Geometry check sheet. Reference: the model listing, model coordinates, mm. A direction names the side the tool comes from. Round coordinates to 2 decimals unless told otherwise and drop trailing zeros. Loops run counter-clockwise (first coordinate to the right, second up) from the corner with the lowest first, then second, coordinate; pieces in that order, holes last. Notation, with made-up numbers: (-5, 82) -> (2, 82) arc R19 ccw to (2, 101) -> close; hole circle Ø5 at (-29.5, 62.25). An arc over 180 degrees is marked (long way). Use a Markdown table: item, result. Add a question column.
Q1. Sectioned sample at A-A, the plane z = 50. Enter the section's corners in (x, y).
Q2. Gauge pin test, flat ends, axial feed: P1, Ø12, axis at x = 16.5, y = -13, coming from the -Z side; P2, Ø12, axis at x = 10.5, y = -11, coming from the +Z side; P3, Ø3.5, axis at x = 19.18, z = 50, coming from the +Y side; P4, Ø8, axis at x = 8.5, z = 10, coming from the -Y side. Record the tip position at first contact, or that the pin passes through.
Q3. Sectioned sample at C-C, the plane y = 3.75. Give the number of separate pieces and of enclosed holes in the cut face, then the cut area to 3 significant figures.
Q4. Set-up check for faces 4 (the face through (21.53, 2.33, 9.69)), 5 (the face through (20.37, 5.46, 29.73)), 6 (the face through (12, -12, 40)), 7 (the face through (12, 0, 10)): record each of +Z, -Z, +X, -X, +Y, -Y from which the full face is reachable in a straight line by a thin tool's end or side.
Q5. Release check for a two-part mould opening along Z. For faces 1 (the face through (3.64, 2.33, 48.12)), 2 (the face through (12, -2, 19)), 3 (the face through (20.37, 5.46, 55.4)) record: released by +Z, released by -Z, zero draft, split by the parting line, or undercut.
Q6. Material ranges on L1, parallel to Z at x = 19.18, y = 5.4; L2, parallel to X at y = 6.4, z = 10; L3, parallel to X at y = 5.25, z = 10, recorded low to high.
Q7. Sectioned sample at B-B, the plane y = -15.75. Enter the section's corners in (x, z).
```python
from build123d import *

# Parameters (mm, degrees)
EXTRUDE_1_DEPTH             = 60
HOLE_WIZARD_M41_D           = 4.5
HOLE_WIZARD_M41_CSINK_D     = 9.4
HOLE_WIZARD_M41_CSINK_ANGLE = 90
EXTRUDE_2_DEPTH             = 24.26
CHAMFER_1_SIZE              = 2.5
CHAMFER_1_SIZE2             = 5
CHAMFER_2_SIZE              = 5
CHAMFER_2_SIZE2             = 2.5


with BuildPart() as part:
    # Эскиз1 → Бобышка-Вытянуть1 (new body)
    with BuildSketch(Plane.XY):
        with BuildLine():
            Line((0.737083196, 7.749967654), (2.429298361, 3.100644699))
            ThreePointArc((2.429298361, 3.100644699), (2.73, 2.890091144), (3.030701639, 3.100644699))
            Line((3.030701639, 3.100644699), (4.722916804, 7.749967654))
            ThreePointArc((4.722916804, 7.749967654), (5.08, 8), (5.437083196, 7.749967654))
            Line((5.437083196, 7.749967654), (7.129298361, 3.100644699))
            ThreePointArc((7.129298361, 3.100644699), (7.43, 2.890091144), (7.730701639, 3.100644699))
            Line((7.730701639, 3.100644699), (9.422916804, 7.749967654))
            ThreePointArc((9.422916804, 7.749967654), (9.78, 8), (10.137083196, 7.749967654))
            Line((10.137083196, 7.749967654), (11.829298361, 3.100644699))
            ThreePointArc((11.829298361, 3.100644699), (12.13, 2.890091144), (12.430701639, 3.100644699))
            Line((12.430701639, 3.100644699), (14.122916804, 7.749967654))
            ThreePointArc((14.122916804, 7.749967654), (14.48, 8), (14.837083196, 7.749967654))
            Line((14.837083196, 7.749967654), (16.529298361, 3.100644699))
            ThreePointArc((16.529298361, 3.100644699), (16.83, 2.890091144), (17.130701639, 3.100644699))
            Line((17.130701639, 3.100644699), (18.822916804, 7.749967654))
            ThreePointArc((18.822916804, 7.749967654), (19.18, 8), (19.537083196, 7.749967654))
            Line((19.537083196, 7.749967654), (21.229298361, 3.100644699))
            ThreePointArc((21.229298361, 3.100644699), (21.53, 2.890091144), (21.830701639, 3.100644699))
            Line((21.830701639, 3.100644699), (23.522916804, 7.749967654))
            ThreePointArc((23.522916804, 7.749967654), (23.945986308, 7.994226946), (24.26, 7.62))
            Line((24.26, 7.62), (24.26, 0))
            Line((24.26, 0), (0, 0))
            Line((0, 0), (0, 7.62))
            ThreePointArc((0, 7.62), (0.314013692, 7.994226946), (0.737083196, 7.749967654))
        make_face()
    extrude(amount=EXTRUDE_1_DEPTH)

    # Зенковка для  винта с плоской головкой M41 (through all)
    with Locations(Plane(origin=(5.08, 0, 50), x_dir=(0, 0, -1), z_dir=(0, -1, 0))):
        with Locations((0, 0), (0, 14.1), (40, 14.1), (40, 0)):
            CounterSinkHole(HOLE_WIZARD_M41_D / 2, HOLE_WIZARD_M41_CSINK_D / 2, counter_sink_angle=HOLE_WIZARD_M41_CSINK_ANGLE)

    # Эскиз6 → Бобышка-Вытянуть2 (add, through all)
    with BuildSketch(Plane.ZY):
        with BuildLine():
            Line((40, -5), (40, -20))
            Line((40, -20), (20, -20))
            Line((20, -20), (20, -5))
            ThreePointArc((20, -5), (18.535533906, -1.464466094), (15, 0))
            Line((15, 0), (45, 0))
            ThreePointArc((45, 0), (41.464466094, -1.464466094), (40, -5))
        make_face()
    extrude(amount=-EXTRUDE_2_DEPTH)

    # Фаска1
    chamfer_1_edges = [part.edges().sort_by_distance(p)[0] for p in [
        (12.13, 0, 0),
    ]]
    chamfer_1_side = [part.faces().sort_by_distance(p)[0] for p in [
        (1.343146193, 5.337937092, 0),
    ]]
    chamfer(chamfer_1_edges, length=CHAMFER_1_SIZE, length2=CHAMFER_1_SIZE2, reference=chamfer_1_side[0])

    # Фаска2
    chamfer_2_edges = [part.edges().sort_by_distance(p)[0] for p in [
        (12.13, 0, 60),
    ]]
    chamfer_2_side = [part.faces().sort_by_distance(p)[0] for p in [
        (12.13, 0, 54.04145744),
    ]]
    chamfer(chamfer_2_edges, length=CHAMFER_2_SIZE, length2=CHAMFER_2_SIZE2, reference=chamfer_2_side[0])


solid = part.part
```
Values:
| question | item | result |
|---|---|---|
| 1 | outline | (0, 0) -> (0.38, 0) -> (2.83, 2.45) -> (2.83, 2.91) arc R0.32 cw to (2.43, 3.1) -> (0.74, 7.75) arc R0.38 ccw to (0, 7.62) -> close; (7.33, 2.45) -> (9.78, 0) -> (14.48, 0) -> (16.93, 2.45) -> (16.93, 2.91) arc R0.32 cw to (16.53, 3.1) -> (14.84, 7.75) arc R0.38 ccw to (14.12, 7.75) -> (12.43, 3.1) arc R0.32 cw to (11.83, 3.1) -> (10.14, 7.75) arc R0.38 ccw to (9.42, 7.75) -> (7.73, 3.1) arc R0.32 cw to (7.33, 2.91) -> close; (21.43, 2.45) -> (23.88, 0) -> (24.26, 0) -> (24.26, 7.62) arc R0.38 ccw to (23.52, 7.75) -> (21.83, 3.1) arc R0.32 cw to (21.43, 2.91) -> close |
| 2 | P1 | z = 20 |
| 2 | P2 | z = 40 |
| 2 | P3 | through |
| 2 | P4 | y = 0 |
| 3 | separate pieces | 10 |
| 3 | enclosed holes | 0 |
| 3 | area | 1,080 mm^2 |
| 4 | face 4 | -Y |
| 4 | face 5 | +Z, -Z, +Y |
| 4 | face 6 | +Z, +X, -X, -Y |
| 4 | face 7 | -Z, +X, -X, -Y |
| 5 | face 1 | undercut |
| 5 | face 2 | released by -Z |
| 5 | face 3 | zero draft |
| 6 | L1 | 0 to 7.75, 12.25 to 47.75, 52.25 to 60 |
| 6 | L2 | 0 to 1.23, 8.93 to 10.63, 13.63 to 15.33, 23.03 to 24.26 |
| 6 | L3 | 0 to 1.65, 8.51 to 11.05, 13.21 to 15.75, 22.61 to 24.26 |
| 7 | outline | (0, 20) -> (24.26, 20) -> (24.26, 40) -> (0, 40) -> close |
